from build123d import *

# Parameters (mm, degrees)
F1_DEPTH    = 25
F2_R        = 3
F3_T1_DEPTH = 47.7014436638
F4_R        = 2


# Not quite as in the source:
# - a fillet or chamfer that OpenCascade refuses, or shapes differently, is made with other operations: its cross-section is extruded or revolved along the edge and cut away or added


with BuildPart() as f1:
    # F0 (on Top) → F1 (new body)
    with BuildSketch(Plane.XY):
        with BuildLine():
            ThreePointArc((10.9601551084, 10.9601551084), (14.3201327539, 5.9315932017), (15.5, 0))
            ThreePointArc((15.5, 0), (-5.9315932017, -14.3201327539), (-10.9601551084, 10.9601551084))
            Line((-10.9601551084, 10.9601551084), (-18.0312229203, 18.0312229203))
            ThreePointArc((-18.0312229203, 18.0312229203), (-9.7584275253, -23.558928079), (25.5, 0))
            ThreePointArc((25.5, 0), (23.558928079, 9.7584275253), (18.0312229203, 18.0312229203))
            Line((18.0312229203, 18.0312229203), (10.9601551084, 10.9601551084))
        make_face()
    extrude(amount=F1_DEPTH)

    # F2
    f2_edges = [f1.edges().sort_by_distance(p)[0] for p in [
        (-18.031223, 18.031223, 12.5),
        (18.031223, 18.031223, 12.5),
    ]]
    fillet(f2_edges, radius=F2_R)

    # F3: chamfer of 5 on 2 edges, made by hand

    # F3_s2 → F3_t1 (cut)
    with BuildSketch(Plane.XY.offset(-11.3507218319)):
        with BuildLine():
            Line((-14.0579159195, 14.0579159195), (-13.3023645022, 7.9559473761))
            ThreePointArc((-13.3023645022, 7.9559473761), (-12.2677824681, 9.4737275301), (-10.9601551084, 10.9601551084))
            Line((-10.9601551084, 10.9601551084), (-14.0579159195, 14.0579159195))
        make_face()
        with BuildLine():
            Line((13.3023645022, 7.9559473761), (14.0579159195, 14.0579159195))
            Line((14.0579159195, 14.0579159195), (10.9601551084, 10.9601551084))
            ThreePointArc((10.9601551084, 10.9601551084), (12.2677824681, 9.4737275301), (13.3023645022, 7.9559473761))
        make_face()
    extrude(amount=F3_T1_DEPTH, mode=Mode.SUBTRACT)

    # F4
    f4_edges = [f1.edges().sort_by_distance(p)[0] for p in [
        (-13.302365, 7.955947, 12.5),
        (-14.057916, 14.057916, 12.5),
        (13.302365, 7.955947, 12.5),
        (14.057916, 14.057916, 12.5),
    ]]
    fillet(f4_edges, radius=F4_R)


solid = f1.part
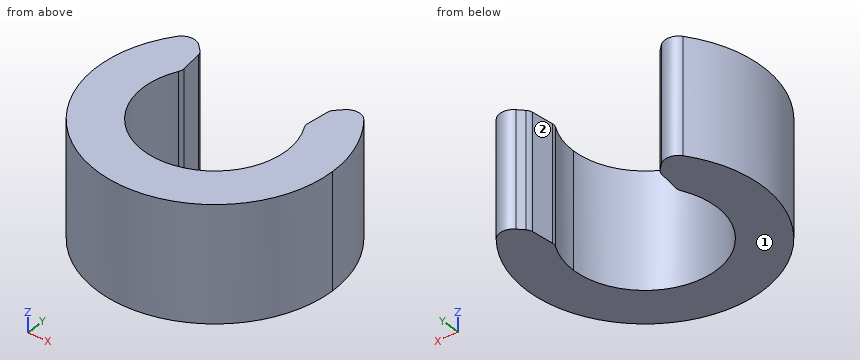
Check sheet for the modelled part. Datum: model origin and axes. Units: mm. Face numbers are marked on the shaded views. A direction names the side the tool comes from. Round coordinates to 2 decimals unless told otherwise and drop trailing zeros. Loops run counter-clockwise (first coordinate to the right, second up) from the corner with the lowest first, then second, coordinate; pieces in that order, holes last.
1. Scan lines: probe 1 along X at (y, z) = (0, 14.75); probe 2 along X at (y, z) = (-8, 9.25); probe 3 along Y at (x, z) = (0, 6.25). Record each from-to range of solid material in increasing order.
2. Set-up check for the marked faces 1 and 2: record each of +Z, -Z, +X, -X, +Y, -Y from which the full face is reachable in a straight line by a thin tool's end or side.
3. Sectioned sample at D-D on y = 12. Record the boundary of the cut face in (x, z), and give its area (3 significant figures).
4. Sectioned sample at B-B on z = 10. Record the boundary of the cut face in (x, y).
5. Sectioned sample at C-C on x = 0. Record the boundary of the cut face in (y, z).
6. Gauge pin test, flat ends, axial feed: pin 1 Ø4 at (y, z) = (-13.5, 14) entering from +X; pin 2 Ø1 at (y, z) = (4.5, 8.5) entering from +X; pin 3 Ø10 at (y, z) = (12.5, 14) entering from +X. Record the tip position at first contact, or that the pin passes through.
7. Sectioned sample at A-A on y = 5.5. Record the boundary of the cut face in (x, z).
Recorded:
1. probe 1: x = -25.5 to -15.5, 15.5 to 25.5
1. probe 2: x = -24.21 to -13.28, 13.28 to 24.21
1. probe 3: y = -25.5 to -15.5
2. face 1: -Z, +X, -X, +Y, -Y
2. face 2: +Z, -Z, +Y
3. outline: (-22.5, 0) - (-13.8, 0) - (-13.8, 25) - (-22.5, 25) - close; (13.8, 0) - (22.5, 0) - (22.5, 25) - (13.8, 25) - close
3. area: 435 mm2
4. outline: (-20.27, 15.47) arc R25.5 ccw (long way) to (20.27, 15.47) arc R3 ccw to (15.77, 15.77) - (14.54, 14.54) arc R2 ccw to (13.97, 13.38) - (13.38, 8.62) arc R2 ccw to (13.61, 7.41) arc R15.5 cw (long way) to (-13.61, 7.41) arc R2 ccw to (-13.38, 8.62) - (-13.97, 13.38) arc R2 ccw to (-14.54, 14.54) - (-15.77, 15.77) arc R3 ccw to start
5. outline: (-25.5, 0) - (-15.5, 0) - (-15.5, 25) - (-25.5, 25) - close
6. pin 1: stops at x = 22.76
6. pin 2: stops at x = 25.18
6. pin 3: stops at x = 24.37
7. outline: (-24.9, 0) - (-14.49, 0) - (-14.49, 25) - (-24.9, 25) - close; (14.49, 0) - (24.9, 0) - (24.9, 25) - (14.49, 25) - close
